CAD build for the part. Positions are in the model's coordinates, mm. Face numbers are marked on the shaded views. A direction names the side the tool comes from. Give positions to 0.01 mm unless a question says otherwise; leave off trailing zeros. Loops run counter-clockwise (first coordinate to the right, second up) from the corner with the lowest first, then second, coordinate; pieces in that order, holes last. Notation, with made-up numbers: (65.25, 50.25) - (115.25, 50.25) arc R22 cw to (115.25, 77.25) - close; hole circle Ø3 at (4.25, 60.5). An arc over 180 degrees is marked (long way). Return JSON: item names as keys, results as strings.
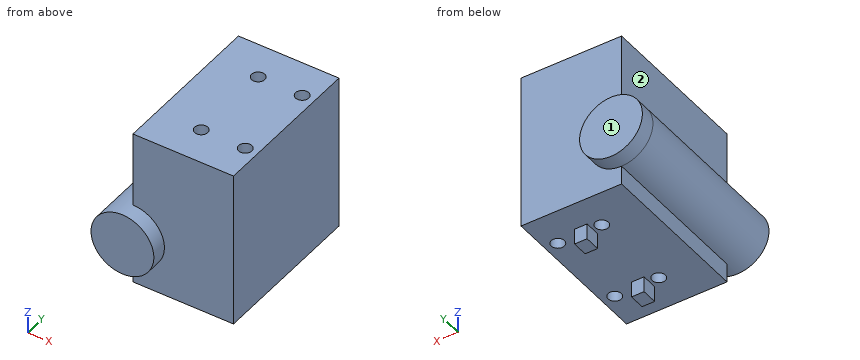
from build123d import *

# Parameters (mm, degrees)
SKETCH001_W       = 32
SKETCH001_H       = 50
PAD_DEPTH         = 50
SKETCH002_W       = 4
SKETCH002_H       = 5
PAD001_DEPTH      = 5
SKETCH003_R       = 2.1
POCKET_DEPTH      = 211.852784
SKETCH004_R       = 10
PAD002_DEPTH      = 5
PAD002_DEPTH_BACK = 55


with BuildPart() as part:
    # Sketch001 → Pad (new body)
    with BuildSketch(Plane.XY):
        Rectangle(SKETCH001_W, SKETCH001_H)
    extrude(amount=PAD_DEPTH)

    # Sketch002 → Pad001 (join)
    with BuildSketch(Plane.XY):
        with Locations((3, 13.5)):
            Rectangle(SKETCH002_W, SKETCH002_H)
        with Locations((3, -13.5)):
            Rectangle(SKETCH002_W, SKETCH002_H)
    extrude(amount=-PAD001_DEPTH)

    # Sketch003 → Pocket (cut, through all)
    with BuildSketch(Plane.XY):
        with Locations((-2, 13.5)):
            Circle(SKETCH003_R)
        with Locations((12, 13.5)):
            Circle(SKETCH003_R)
    pocket = extrude(amount=POCKET_DEPTH, mode=Mode.SUBTRACT)

    # Mirrored: Pocket across Sketch003 H_Axis
    add(pocket.mirror(Plane.ZX), mode=Mode.SUBTRACT)

    # Sketch004 (on DatumPlane) → Pad002 (join, two sides)
    with BuildSketch(Plane(origin=(0, 25, 0), x_dir=(-1, 0, 0), z_dir=(0, 1, 0))) as pad002_sk:
        with Locations((16, 16)):
            Circle(SKETCH004_R)
    extrude(amount=PAD002_DEPTH)
    extrude(pad002_sk.sketch, amount=-PAD002_DEPTH_BACK)


solid = part.part
1. Cut at A-A, the plane x = -2. Write the cut outline in (y, z).
Values follow:
{"outline": "(-25, 0) - (-15.6, 0) - (-15.6, 50) - (-25, 50) - close; (-11.4, 0) - (11.4, 0) - (11.4, 50) - (-11.4, 50) - close; (15.6, 0) - (25, 0) - (25, 50) - (15.6, 50) - close"}
2. Cut at C-C, the plane z = 30. Write the cut outline in (x, y), plus the area to 3 significant figures.
Values follow:
{"outline": "(-16, -25) - (16, -25) - (16, 25) - (-16, 25) - close; hole circle Ø4.2 at (-2, -13.5); hole circle Ø4.2 at (-2, 13.5); hole circle Ø4.2 at (12, -13.5); hole circle Ø4.2 at (12, 13.5)", "area": "1,540 mm²"}
3. Drop flat-ended pins along their axis: P1, Ø4, axis at x = 12, y = 13.5, coming from the +Z side; P2, Ø12, axis at x = 8, z = 2, coming from the -Y side; P3, Ø2.5, axis at y = 14.5, z = -2, coming from the +X side; P4, Ø8, axis at y = 5.5, z = 20.5, coming from the -X side. Give the stop position or say it passes through.
Values follow:
{"P1": "passes through", "P2": "stops at y = -25", "P3": "stops at x = 5", "P4": "stops at x = -25.99"}
4. Drill centre lines: probe 1 along Y at (x, z) = (-2, 15); probe 2 along X at (y, z) = (13.5, 33); probe 3 along X at (y, z) = (-13.5, 25). Where is each one in solid material? Low to high.
Values follow:
{"probe 1": "y = -25 to -15.6, -11.4 to 11.4, 15.6 to 25", "probe 2": "x = -16 to -4.1, 0.1 to 9.9, 14.1 to 16", "probe 3": "x = -20.36 to -4.1, 0.1 to 9.9, 14.1 to 16"}
5. Cut at B-B, the plane y = -13.5. Write the cut outline in (x, z).
Values follow:
{"outline": "(-16, 0) - (-4.1, 0) - (-4.1, 50) - (-16, 50) - (-16, 26) arc R10 ccw to (-16, 6) - close; (0.1, 0) - (1, 0) - (1, -5) - (5, -5) - (5, 0) - (9.9, 0) - (9.9, 50) - (0.1, 50) - close; (14.1, 0) - (16, 0) - (16, 50) - (14.1, 50) - close"}
6. Cut at D-D, the plane x = 2.5. Write the cut outline in (y, z).
Values follow:
{"outline": "(-25, 0) - (-16, 0) - (-16, -5) - (-11, -5) - (-11, 0) - (11, 0) - (11, -5) - (16, -5) - (16, 0) - (25, 0) - (25, 50) - (-25, 50) - close"}
7. Which spindle directions (+Z, -Z, +X, -X, +Y, -Y) get a long thin tool onto all of the face, cutting with end or side? Do the marked faces 1 and 2. Say none if no direction does.
Values follow:
{"face 1": "+Z, -Z, +X, -X, +Y", "face 2": "+Z, -X, +Y, -Y"}
